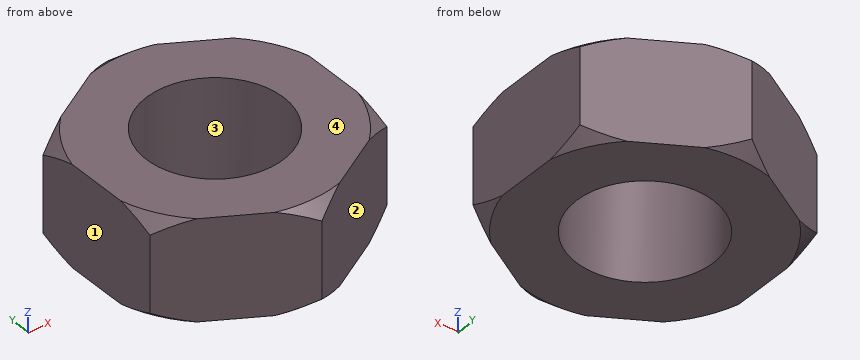
from build123d import *

# Parameters (mm, degrees)
SKETCH_R  = 1.5
PAD_DEPTH = 1.1


with BuildPart() as body001:
    # Sketch002 → Revolution (revolve)
    with BuildSketch(Plane.YZ):
        Polygon((2.1, 1.6), (3.1, 0.75), (3.1, -0.75), (2.1, -1.6), (4.1, -1.6), (4.1, 1.6), align=None)
    revolve(axis=Axis((0, 0, 0), (0, 0, 1)))


with BuildPart() as cut:
    # Sketch → Pad (new body, symmetric)
    with BuildSketch(Plane.XY):
        Polygon((2.6, 1.501111), (0, 3.002221), (-2.6, 1.501111), (-2.6, -1.501111), (0, -3.002221), (2.6, -1.501111), align=None)
        Circle(SKETCH_R, mode=Mode.SUBTRACT)
    extrude(amount=PAD_DEPTH, both=True)

    # Cut: cut Body001
    add(body001.part, mode=Mode.SUBTRACT)


solid = cut.part
The listing builds one solid part. Answer for the finished solid, in the listing's coordinates (mm). Face numbers are marked on the shaded views. Give positions to 0.01 mm unless a question says otherwise; leave off trailing zeros. Order: outer loops, then holes, each group sorted by start corner. A loop starts at its lowest first (then second) coordinate and runs counter-clockwise, first axis right, second up. Notation, with made-up numbers: (14, 19) - (49, 19) arc R35 cw to (49, 53) - close; hole circle Ø10 at (11, 74). An arc over 180 degrees is marked (long way). Use one line per item in the form item = value.
1) This flat-tipped pin is pushed along its axis until it touches: pin 1 (1 mm diameter, centred on x = -2, z = -1, fed in from +Y). Where does it stop, or does it pass through?
Verdict:
pin_1 = 2.14
2) Consider probe 1 along Y at (x, z) = (0.8, -0.15); probe 2 along Y at (x, z) = (1.1, 0.3); probe 3 along X at (y, z) = (-2.5, 0). Determine where each line is inside the solid, lowest interval first. Write a range as [from, to].
Verdict:
probe_1 = [-2.54, -1.27], [1.27, 2.54]
probe_2 = [-2.37, -1.02], [1.02, 2.37]
probe_3 = [-0.87, 0.87]
3) The mould has two halves that part along X. Classify the marked faces 1, 2, 3 and 4: released by +X, released by -X, zero draft, split by the parting line, or undercut.
Verdict:
face_1 = released by -X
face_2 = released by +X
face_3 = undercut
face_4 = zero draft
4) Find section C-C on x = 1.75. Determine the outline of the cut face in (y, z), and give its area (3 significant figures).
Verdict:
outline = (-1.99, -1.1) - (1.99, -1.1) - (1.99, 1.1) - (-1.99, 1.1) - close
area = 8.76 mm^2
5) Find section B-B on y = 0. Determine the outline of the cut face in (x, z), and give its area (3 significant figures).
Verdict:
outline = (-2.6, -1.1) - (-1.5, -1.1) - (-1.5, 1.1) - (-2.6, 1.1) - close; (1.5, -1.1) - (2.6, -1.1) - (2.6, 1.1) - (1.5, 1.1) - close
area = 4.84 mm^2
6) Find section A-A on z = 0. Determine the outline of the cut face in (x, y).
Verdict:
outline = (-2.6, -1.5) - (0, -3) - (2.6, -1.5) - (2.6, 1.5) - (0, 3) - (-2.6, 1.5) - close; hole circle Ø3 at (0, 0)
